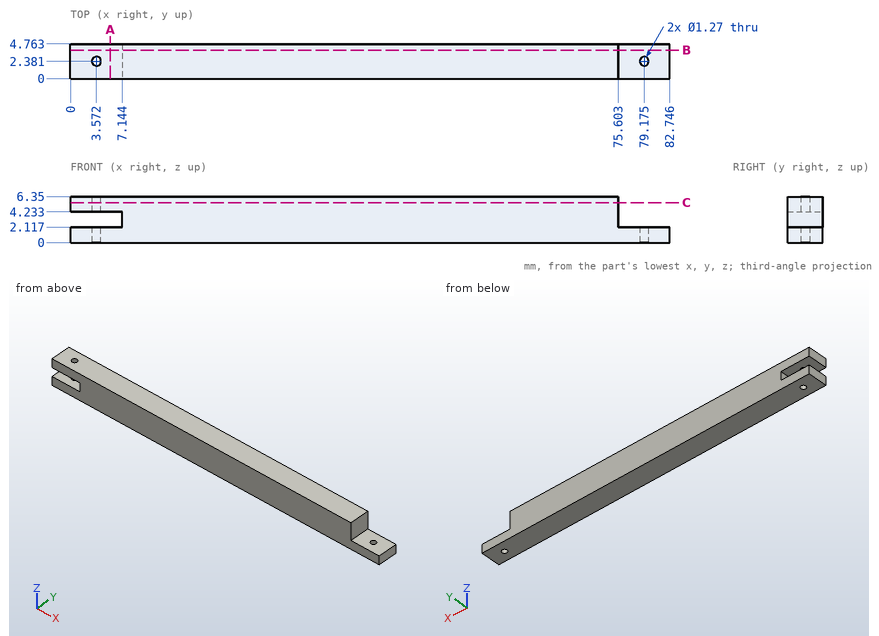
Can you work these out from the drawing? Everything is in mm from the part's minimum corner. Coordinates: 2 decimals unless noted, no trailing zeros. Order: outer loops, then holes, each group sorted by start corner. A loop starts at its lowest first (then second) coordinate and runs counter-clockwise, first axis right, second up. Notation, with made-up numbers: (-25.5, -40) -> (25.5, -40) arc R16 cw to (25.5, -16) -> close; hole circle Ø7 at (83.5, 65). An arc over 180 degrees is marked (long way). Return JSON: item names as keys, results as strings.
1) If we section it at C-C on z = 5.5: List the corners of the cut face in (x, y) for me (1 decimal).
Conclusion:
{"outline": "(0, 0) -> (75.6, 0) -> (75.6, 4.8) -> (0, 4.8) -> close; hole circle Ø1.3 at (3.6, 2.4)"}
2) I'm going to push flat-ended pins straight in: P1, Ø1.5, axis at x = 3.57, y = 2.38, coming from the +Z side; P2, Ø1.7, axis at y = 2.5, z = 3, coming from the -X side. Where does each tip first touch, or does it pass through?
Conclusion:
{"P1": "stops at z = 6.35", "P2": "stops at x = 7.14"}
3) If we section it at A-A on x = 5.5: List the corners of the cut face in (y, z) for me.
Conclusion:
{"outline": "(0, 0) -> (4.76, 0) -> (4.76, 2.12) -> (0, 2.12) -> close; (0, 4.23) -> (4.76, 4.23) -> (4.76, 6.35) -> (0, 6.35) -> close"}
4) If I drill on probe 1 along X at (y, z) = (2.05, 1.25) (1 decimal); probe 2 along X at (y, z) = (4.1, 6); probe 3 along X at (y, z) = (3.8, 4), over which ranges is the centre line in solid material (lowest first)?
Conclusion:
{"probe 1": "x = 0 to 3, 4.1 to 78.6, 79.7 to 82.7", "probe 2": "x = 0 to 75.6", "probe 3": "x = 7.14 to 75.6"}
5) If we section it at B-B on y = 3.9: List the corners of the cut face in (x, z) for me, plus the area to 3 significant figures.
Conclusion:
{"outline": "(0, 0) -> (82.75, 0) -> (82.75, 2.12) -> (75.6, 2.12) -> (75.6, 6.35) -> (0, 6.35) -> (0, 4.23) -> (7.14, 4.23) -> (7.14, 2.12) -> (0, 2.12) -> close", "area": "480 mm²"}
